from build123d import *

# Parameters (mm, degrees)
SKETCH1_W               = 40
SKETCH1_H               = 32
BOSS_EXTRUDE1_DEPTH     = 17
SKETCH3_W               = 31
SKETCH3_H               = 19.5
BOSS_EXTRUDE2_DEPTH     = 5.5
CUT_EXTRUDE1_REACH      = 93.662
SKETCH2_R               = 1.75
CUT_EXTRUDE2_DEPTH      = 6
CUT_EXTRUDE2_DEPTH_BACK = 6
SKETCH5_R               = 2.5
CUT_EXTRUDE3_DEPTH      = 21.5
SKETCH6_R               = 11.75
CUT_EXTRUDE4_DEPTH      = 22.5
CUT_EXTRUDE5_DEPTH      = 7
CUT_EXTRUDE5_DEPTH_BACK = 7
SKETCH9_R               = 3
CUT_EXTRUDE7_DEPTH      = 13
SKETCH10_R              = 3
CUT_EXTRUDE8_DEPTH      = 18.5
CUT_EXTRUDE6_REACH      = 79.599


with BuildPart() as part:
    # Sketch1 → Boss-Extrude1 (new body)
    with BuildSketch(Plane.XY):
        with Locations((-41.344294363, 48.285102326)):
            Rectangle(SKETCH1_W, SKETCH1_H)
    extrude(amount=BOSS_EXTRUDE1_DEPTH)

    # Sketch3 → Boss-Extrude2 (add)
    with BuildSketch(Plane(origin=(0, 0, 0), x_dir=(-1, 0, 0), z_dir=(0, 0, -1))):
        with Locations((36.844294363, 54.535102326)):
            Rectangle(SKETCH3_W, SKETCH3_H)
    extrude(amount=BOSS_EXTRUDE2_DEPTH)

    # Cut-Extrude1: up to this face of the body (flat: up to its plane)
    cut_extrude1_end = Plane(part.part.faces().sort_by_distance((-36.844294363, 54.535102326, -5.5))[0])
    # Sketch2 → Cut-Extrude1 (cut, up to the picked face)
    with BuildSketch(Plane.XY.offset(17), mode=Mode.PRIVATE) as cut_extrude1_sk1:
        with Locations((-27.344294363, 60.785102326)):
            Circle(SKETCH2_R)
    cut_extrude1_tool1 = split(extrude(cut_extrude1_sk1.sketch, amount=-CUT_EXTRUDE1_REACH, mode=Mode.PRIVATE), bisect_by=cut_extrude1_end, keep=Keep.BOTH, mode=Mode.PRIVATE)
    # Sketch2 → Cut-Extrude1 (cut, up to the picked face)
    with BuildSketch(Plane.XY.offset(17), mode=Mode.PRIVATE) as cut_extrude1_sk2:
        with Locations((-27.344294363, 38.285102326)):
            Circle(SKETCH2_R)
    cut_extrude1_tool2 = split(extrude(cut_extrude1_sk2.sketch, amount=-CUT_EXTRUDE1_REACH, mode=Mode.PRIVATE), bisect_by=cut_extrude1_end, keep=Keep.BOTH, mode=Mode.PRIVATE)
    # Sketch2 → Cut-Extrude1 (cut, up to the picked face)
    with BuildSketch(Plane.XY.offset(17), mode=Mode.PRIVATE) as cut_extrude1_sk3:
        with Locations((-53.344294363, 38.285102326)):
            Circle(SKETCH2_R)
    cut_extrude1_tool3 = split(extrude(cut_extrude1_sk3.sketch, amount=-CUT_EXTRUDE1_REACH, mode=Mode.PRIVATE), bisect_by=cut_extrude1_end, keep=Keep.BOTH, mode=Mode.PRIVATE)
    add(cut_extrude1_tool1.solids().sort_by(Axis((-27.344294, 60.785102, 17), (0, 0, -1)))[0], mode=Mode.SUBTRACT)
    add(cut_extrude1_tool2.solids().sort_by(Axis((-27.344294, 38.285102, 17), (0, 0, -1)))[0], mode=Mode.SUBTRACT)
    add(cut_extrude1_tool3.solids().sort_by(Axis((-53.344294, 38.285102, 17), (0, 0, -1)))[0], mode=Mode.SUBTRACT)

    # Sketch4 → Cut-Extrude2 (cut, two sides: drawn at the far end of the back side and taken through both)
    with BuildSketch(Plane(origin=(-40.344294363, 0, 0), x_dir=(0, 0, -1), z_dir=(1, 0, 0)).offset(-CUT_EXTRUDE2_DEPTH_BACK)):
        with BuildLine():
            Line((0.5, 57.284133416), (11.5, 57.284133416))
            Line((11.5, 57.284133416), (11.5, 46.284133416))
            ThreePointArc((11.5, 46.284133416), (-7.278174593, 38.505958823), (0.5, 57.284133416))
        make_face()
    extrude(amount=CUT_EXTRUDE2_DEPTH + CUT_EXTRUDE2_DEPTH_BACK, mode=Mode.SUBTRACT)

    # Sketch5 → Cut-Extrude3 (cut)
    with BuildSketch(Plane(origin=(0, 0, -5.5), x_dir=(-1, 0, 0), z_dir=(0, 0, -1))):
        with Locations((40.344294363, 46.284133416)):
            Circle(SKETCH5_R)
    extrude(amount=-CUT_EXTRUDE3_DEPTH, mode=Mode.SUBTRACT)

    # Sketch6 → Cut-Extrude4 (cut)
    with BuildSketch(Plane.XY.offset(17)):
        with Locations((-68.344294363, 61.785102326)):
            Circle(SKETCH6_R)
    extrude(amount=-CUT_EXTRUDE4_DEPTH, mode=Mode.SUBTRACT)

    # Sketch7 → Cut-Extrude5 (cut, two sides: drawn at the far end of the back side and taken through both)
    with BuildSketch(Plane(origin=(-40.344294363, 0, 0), x_dir=(0, 0, -1), z_dir=(1, 0, 0)).offset(-CUT_EXTRUDE5_DEPTH_BACK)):
        with BuildLine():
            Line((0.5, 50.784133416), (3.5, 50.784133416))
            ThreePointArc((3.5, 50.784133416), (8, 46.284133416), (3.5, 41.784133416))
            Line((3.5, 41.784133416), (0.5, 41.784133416))
            ThreePointArc((0.5, 41.784133416), (-4, 46.284133416), (0.5, 50.784133416))
        make_face()
    extrude(amount=CUT_EXTRUDE5_DEPTH + CUT_EXTRUDE5_DEPTH_BACK, mode=Mode.SUBTRACT)

    # Sketch9 → Cut-Extrude7 (cut)
    with BuildSketch(Plane.XY.offset(17)):
        with Locations((-27.344294363, 38.285102326)):
            Circle(SKETCH9_R)
        with Locations((-53.344294363, 38.285102326)):
            Circle(SKETCH9_R)
    extrude(amount=-CUT_EXTRUDE7_DEPTH, mode=Mode.SUBTRACT)

    # Sketch10 → Cut-Extrude8 (cut)
    with BuildSketch(Plane.XY.offset(17)):
        with Locations((-27.344294363, 60.785102326)):
            Circle(SKETCH10_R)
    extrude(amount=-CUT_EXTRUDE8_DEPTH, mode=Mode.SUBTRACT)

    # Cut-Extrude6: up to this face of the body (flat: up to its plane)
    cut_extrude6_end = Plane(part.part.faces().sort_by_distance((-61.344294363, 42.316455804, 8.5))[0])
    # Sketch8 → Cut-Extrude6 (cut, up to the picked face)
    with BuildSketch(Plane(origin=(-21.344294363, 0, 0), x_dir=(0, 0, -1), z_dir=(1, 0, 0)), mode=Mode.PRIVATE) as cut_extrude6_sk1:
        with BuildLine():
            Line((-9.261769408, 67.698643379), (-19.68345764, 67.698643379))
            Line((-19.68345764, 67.698643379), (-19.68345764, 31.088127449))
            Line((-19.68345764, 31.088127449), (-13.3551738, 31.088127449))
            ThreePointArc((-13.3551738, 31.088127449), (-16.792545144, 50.006557071), (-9.261769408, 67.698643379))
        make_face()
    cut_extrude6_tool1 = split(extrude(cut_extrude6_sk1.sketch, amount=-CUT_EXTRUDE6_REACH, mode=Mode.PRIVATE), bisect_by=cut_extrude6_end, keep=Keep.BOTH, mode=Mode.PRIVATE)
    add(cut_extrude6_tool1.solids().sort_by(Axis((-21.344294, 51.901758, 16.96141), (-1, 0, 0)))[0], mode=Mode.SUBTRACT)


solid = part.part
CAD build for the part. Positions are in the model's coordinates, mm. A direction names the side the tool comes from. Round coordinates to 2 decimals unless told otherwise and drop trailing zeros. Loops run counter-clockwise (first coordinate to the right, second up) from the corner with the lowest first, then second, coordinate; pieces in that order, holes last.
(1) Cut at B-B (x = -40.5). Give the cut face in (y, z).
(2) Cut at D-D (z = 9.25). Give the cut face in (x, y), plus the area to 3 significant figures.
(3) Which spindle directions (+Z, -Z, +X, -X, +Y, -Y) get a long thin tool onto all of the face, cutting with end or side? Do faces 5 (the cylindrical face through (-27.73, 41.26, 10.4)), 6 (the flat face through (-40, 57.284, -3)), 7 (the flat face through (-52.344, 54, -3)). Say none if no direction does.
(4) Two-plate mould, pull along X, no slides. Class faces 1 (the flat face through (-21.344, 48, 6)), 2 (the flat face through (-51, 38, 4)), 3 (the flat face through (-47.344, 47, -1)), 4 (the flat face through (-42, 32.285, 7)): +X half, -X half, draft (parallel to the pull), parting line (faces both ways), or undercut.
(5) Cut at C-C (y = 51.5). Give the cut face in (x, z).
(6) Wall check: line 1 along Y through (x, z) = (-28, 11.25); line 2 along X through (y, z) = (51.5, -1); line 3 along Y through (x, z) = (-29.5, 7.25). Give the ranges that are in metal, low to high.
(7) Drop flat-ended pins along their axis: pin 1 (8 mm diameter, centred on x = -40.34, y = 46.28, fed in from -Z); pin 2 (5.5 mm diameter, centred on x = -53.34, y = 38.29, fed in from -Z); pin 3 (3 mm diameter, centred on x = -28, y = 61.5, fed in from +Z). Give the stop position or say it passes through.
(8) Cut at A-A (z = 1.5). Give the cut face in (x, y), plus the area to 3 significant figures.
Findings below:
1. outline: (32.29, 0) - (35.3, 0) arc R11 cw to (43.79, 10.21) - (43.79, 16) - (48.78, 16) - (48.78, 10.21) arc R11 cw to (57.28, -0.5) - (57.28, -5.5) - (64.29, -5.5) - (64.29, 11.75) arc R33.5 ccw to (32.29, 13.93) - close
2. outline: (-61.34, 32.29) - (-21.34, 32.29) - (-21.34, 64.29) - (-56.86, 64.29) arc R11.75 cw to (-61.34, 52.35) - close; hole circle Ø6 at (-53.34, 38.29); hole (-46.34, 41.19) - (-34.34, 41.19) - (-34.34, 51.38) - (-46.34, 51.38) - close; hole circle Ø6 at (-27.34, 38.29); hole circle Ø6 at (-27.34, 60.79)
2. area: 1,030 mm2
3. face 5: +Z
3. face 6: -Z, -Y
3. face 7: -Z, -X, +Y, -Y
4. face 1: +X half
4. face 2: undercut
4. face 3: undercut
4. face 4: draft
5. outline: (-61.34, 0) - (-52.34, 0) - (-52.34, -5.5) - (-46.34, -5.5) - (-46.34, 9.18) - (-34.34, 9.18) - (-34.34, -5.5) - (-21.34, -5.5) - (-21.34, 16.59) - (-61.34, 16.59) - close
6. line 1: y = 32.29 to 35.36, 41.21 to 57.86, 63.71 to 64.29
6. line 2: x = -52.34 to -46.34, -34.34 to -21.34
6. line 3: y = 32.29 to 36.2, 40.37 to 58.7, 62.87 to 64.29
7. pin 1: stops at z = 9.75
7. pin 2: stops at z = 0
7. pin 3: stops at z = -1.5
8. outline: (-61.34, 32.29) - (-21.34, 32.29) - (-21.34, 64.29) - (-56.86, 64.29) arc R11.75 cw to (-61.34, 52.35) - close; hole circle Ø3.5 at (-53.34, 38.29); hole (-47.34, 42.25) - (-46.34, 42.25) - (-46.34, 35.47) - (-34.34, 35.47) - (-34.34, 42.25) - (-33.34, 42.25) - (-33.34, 50.32) - (-34.34, 50.32) - (-34.34, 57.1) - (-46.34, 57.1) - (-46.34, 50.32) - (-47.34, 50.32) - close; hole circle Ø6 at (-27.34, 60.79); hole circle Ø3.5 at (-27.34, 38.29)
8. area: 914 mm2
